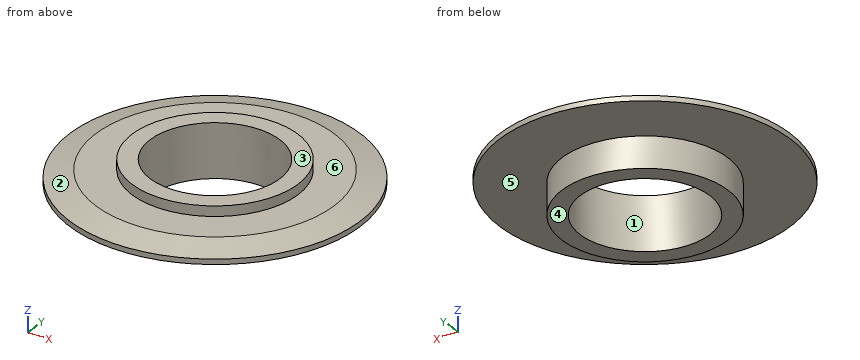
Autodesk Inventor part; units mm, degrees
ref_plane "YZ Plane" through (0, 0, 0) normal (1, 0, 0) x (0, 1, 0)
ref_plane "XZ Plane" through (0, 0, 0) normal (0, 1, 0) x (-1, 0, 0)
ref_plane "XY Plane" through (0, 0, 0) normal (0, 0, 1) x (1, 0, 0)
sketch "草圖1" plane through (0, 0, 0) normal (0, 0, 1) x (1, 0, 0)
  circle A0 centre (0, 0) radius 16
extrude "擠出1" add sketch "草圖1" along normal blind 6
sketch "草圖2" plane through (0, 0, 6) normal (0, 0, 1) x (1, 0, 0)
  circle A0 centre (0, 0) radius 28
extrude "擠出2" add sketch "草圖2" along normal blind 2.4
sketch "草圖3" plane through (0, 0, 8.4) normal (0, 0, 1) x (1, 0, 0)
  circle A0 centre (0, 0) radius 16
extrude "擠出3" add sketch "草圖3" along normal blind 1.95
hole "孔1" at (0, 0, 10.35) direction (0, 0, -1) diameter 25 end through all
chamfer "倒角1" distance 1.4 distance2 5 1 edges at (-28, 0, 8.4) measured on face at (27.9092, -2.2531, 7.6)
properties part number "KL-SL-023-KMB-601-PT"
Geometry check sheet. Reference: the model listing, model coordinates, mm. Face numbers are marked on the shaded views. A direction names the side the tool comes from. Coordinates: 2 decimals unless noted, no trailing zeros. Loops run counter-clockwise (first coordinate to the right, second up) from the corner with the lowest first, then second, coordinate; pieces in that order, holes last. Notation, with made-up numbers: (-18.5, 76) - (35.5, 76) arc R17 ccw to (35.5, 106) - close; hole circle Ø6 at (75, 40). An arc over 180 degrees is marked (long way). One line per item, written item: value. Start each with the question number.
(1) Mould release check, pull along Y, two halves, no side actions. Record for the marked faces 1, 2 and 3: released by +Y, released by -Y, zero draft, split by the parting line, or undercut.
(2) Tool access check on the marked faces 4, 5 and 6. Record the directions out of +Z, -Z, +X, -X, +Y, -Y that give a thin tool (end or side, any length) a straight path to the whole face; none if there is none.
(3) Cross-section at C-C on z = 2.25. Enter the section's corners in (x, y).
(4) Cross-section at A-A on x = 0. Enter the section's corners in (y, z).
(5) Depth check by flat-ended pin: P1, Ø12, axis at x = 3.5, y = -3.5, coming from the -Z side; P2, Ø6, axis at x = 1.5, z = 7, coming from the -Y side; P3, Ø2, axis at x = 0, y = 20.5, coming from the +Z side; P4, Ø1.5, axis at x = 14.5, z = 2.5, coming from the -Y side. Enter the tip coordinate at first touch or a pass-through.
(6) Material ranges on line 1 (Y direction, x = 0, z = 5.75); line 2 (Z direction, x = -17.5, y = 14.5); line 3 (Y direction, x = 3, z = 6.75), recorded low to high. Write a range as [from, to].
Results below:
1. face 1: undercut
1. face 2: split by the parting line
1. face 3: zero draft
2. face 4: -Z, +X, -X, +Y, -Y
2. face 5: -Z
2. face 6: +Z
3. outline: circle Ø32 at (0, 0); hole circle Ø25 at (0, 0)
4. outline: (-28, 6) - (-16, 6) - (-16, 0) - (-12.5, 0) - (-12.5, 10.35) - (-16, 10.35) - (-16, 8.4) - (-23, 8.4) - (-28, 7) - close; (12.5, 0) - (16, 0) - (16, 6) - (28, 6) - (28, 7) - (23, 8.4) - (16, 8.4) - (16, 10.35) - (12.5, 10.35) - close
5. P1: passes through
5. P2: stops at y = -28
5. P3: stops at z = 8.4
5. P4: stops at y = -8.18
6. line 1: y = [-16, -12.5], [12.5, 16]
6. line 2: z = [6, 8.4]
6. line 3: y = [-27.84, -12.13], [12.13, 27.84]
